```python
from build123d import *

# Parameters (mm, degrees)
SKETCH4_R = 6.35


with BuildPart() as part:
    # Sweep3: sweep along a path in Sketch5
    with BuildLine(Plane.XY) as sweep3_path:
        Line((0, 0), (31.75, 0))
        Line((31.75, 0), (58.62223186, 152.4))
        Line((58.62223186, 152.4), (90.37223186, 152.4))
        Line((90.37223186, 152.4), (120.549008468, 152.4))
        Line((120.549008468, 152.4), (147.421240328, 304.8))
        Line((147.421240328, 304.8), (181.551345013, 304.8))
    # Sketch4 → Sweep3 (sweep)
    with BuildSketch(Plane(origin=(0, 0, 0), x_dir=(0, 0, -1), z_dir=(1, 0, 0))):
        Circle(SKETCH4_R)
    sweep(path=sweep3_path.line, transition=Transition.RIGHT)


solid = part.part
```
Source: CAD feature listing. Evaluate the final solid. Frame: model axes, mm. A direction names the side the tool comes from. Coordinates: 2 decimals unless noted, no trailing zeros. Write each loop counter-clockwise with the first axis right and the second up, starting at its lowest first coordinate (ties: lowest second). Pieces come first, ordered by that corner, then holes. Notation, with made-up numbers: (75.25, 67) - (109.25, 67) arc R29 ccw to (109.25, 90) - close; hole circle Ø8 at (14, -3). An arc over 180 degrees is marked (long way). Answer as a JSON object with one key per item and string values.
Q1. Section query B-B, the plane x = 68. Output: boundary loops of the cut face in (y, z).
Ans:
{"outline": "circle Ø12.7 at (152.4, 0)"}
Q2. Set-up query: faces 1 (the cylindrical face through (90.094, 154.307, -6.057)), 2 (the cylindrical face through (166.5, 311.1, 0.8)), 3 (the flat face through (181.551, 305, 0)), 4 (the cylindrical face through (14.68, -6.2, 1.38)). Return all of +Z, -Z, +X, -X, +Y, -Y with unobstructed straight access to the full face (end or side cutting, diameter ignored); none if empty.
Ans:
{"face 1": "none", "face 2": "+X", "face 3": "+Z, -Z, +X, +Y, -Y", "face 4": "-X"}
Q3. First-contact query: pin 1 Ø5 at (y, z) = (48, -2) entering from +X; pin 2 Ø4 at (y, z) = (184.5, -4) entering from -X; pin 3 Ø6 at (y, z) = (229.5, -2) entering from -X. Flat tips, straight axial feed; report the tip coordinate or a pass-through.
Ans:
{"pin 1": "stops at x = 47", "pin 2": "stops at x = 120.01", "pin 3": "stops at x = 127.26"}
Q4. Material intervals for line 1 (Z direction, x = 130.5, y = 211); line 2 (X direction, y = 42, z = -1); line 3 (X direction, y = 176, z = 3.5), sorted ascending. Write a range as [from, to].
Ans:
{"line 1": "z = [-6.34, 6.34]", "line 2": "x = [32.79, 45.52]", "line 3": "x = [119.33, 130.09]"}
Q5. Section query A-A, the plane z = 0. Output: boundary loops of the cut face in (x, y), plus the area to 3 significant figures.
Ans:
{"outline": "(0, -6.35) - (37.08, -6.35) - (63.95, 146.05) - (125.88, 146.05) - (152.75, 298.45) - (181.55, 298.45) - (181.55, 311.15) - (142.09, 311.15) - (115.22, 158.75) - (53.29, 158.75) - (26.42, 6.35) - (0, 6.35) - close", "area": "5,550 mm2"}
